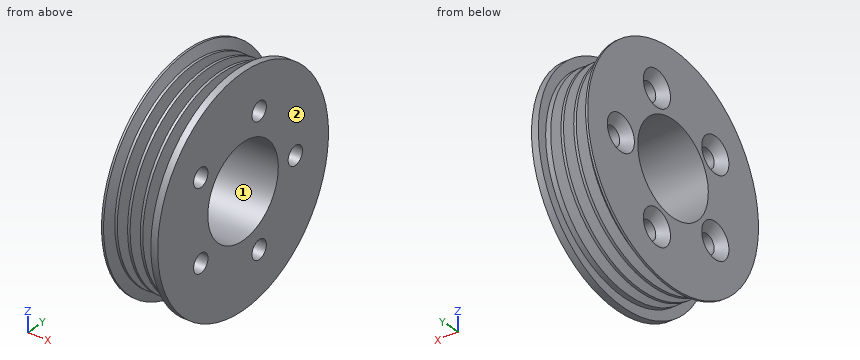
```python
from build123d import *

# Parameters (mm, degrees)
ESCAREADO_PARA_PARAFUSO_COM_CABE_A_ESCAR_D           = 5.5
ESCAREADO_PARA_PARAFUSO_COM_CABE_A_ESCAR_CSINK_D     = 10.4
ESCAREADO_PARA_PARAFUSO_COM_CABE_A_ESCAR_CSINK_ANGLE = 90
PADR_OCIRCULAR1_COUNT                                = 5
ESBO_O5_R                                            = 32.7
ESBO_O5_R_2                                          = 13.5
ESBO_O5_R_3                                          = 2.75
RESSALTO_EXTRUS_O1_DEPTH                             = 2


with BuildPart() as part:
    # Esboço1 → Revolução1 (revolve)
    with BuildSketch(Plane.XY, mode=Mode.PRIVATE) as revolu_o1_sk:
        Polygon((0, 13.5), (16.5, 13.5), (16.5, 29.9), (13, 29.9), (11.9, 24.9), (11.1, 24.9), (10, 29.9), (9.25, 29.9), (8.15, 24.9), (7.35, 24.9), (6.25, 29.9), (5.5, 29.9), (4.4, 24.9), (3.6, 24.9), (2.5, 29.9), (0, 29.9), align=None)
    revolve(revolu_o1_sk.sketch.rotate(Axis((0, 0, 0), (1, 0, 0)), 90), axis=Axis((0, 0, 0), (1, 0, 0)))

    # Escareado para parafuso com cabeça escareada elevada de M51 (through all)
    with Locations(Plane.ZY):
        with Locations((0, 20)):
            escareado_para_parafuso_com_cabe_a_escar = CounterSinkHole(ESCAREADO_PARA_PARAFUSO_COM_CABE_A_ESCAR_D / 2, ESCAREADO_PARA_PARAFUSO_COM_CABE_A_ESCAR_CSINK_D / 2, counter_sink_angle=ESCAREADO_PARA_PARAFUSO_COM_CABE_A_ESCAR_CSINK_ANGLE)

    # PadrãoCircular1: Escareado para parafuso com cabeça escareada elevada de M51 ×5 about axis
    padr_ocircular1_axis = Axis((0, 0, 0), (1, 0, 0))
    for i in range(1, PADR_OCIRCULAR1_COUNT):
        add(escareado_para_parafuso_com_cabe_a_escar.rotate(padr_ocircular1_axis, i * 360 / PADR_OCIRCULAR1_COUNT), mode=Mode.SUBTRACT)

    # Esboço4 → Revolução2 (revolve)
    with BuildSketch(Plane.XY, mode=Mode.PRIVATE) as revolu_o2_sk:
        Polygon((0, 29.9), (0, 32.7), (0.6, 32.7), (1.75, 29.9), align=None)
    revolve(revolu_o2_sk.sketch.rotate(Axis((0, 0, 0), (1, 0, 0)), 90), axis=Axis((0, 0, 0), (1, 0, 0)))

    # Esboço5 → Ressalto-extrusão1 (add)
    with BuildSketch(Plane(origin=(16.5, 0, 0), x_dir=(0, 0, -1), z_dir=(1, 0, 0))):
        with Locations(Location((0, 0, 0), (0, 0, 180))):
            Circle(ESBO_O5_R)
        with Locations(Location((0, 0, 0), (0, 0, 180))):
            Circle(ESBO_O5_R_2, mode=Mode.SUBTRACT)
        with Locations(Location((-11.755705046, -16.180339887, 0), (0, 0, 180))):
            Circle(ESBO_O5_R_3, mode=Mode.SUBTRACT)
        with Locations(Location((11.755705046, -16.180339887, 0), (0, 0, 180))):
            Circle(ESBO_O5_R_3, mode=Mode.SUBTRACT)
        with Locations(Location((19.021130326, 6.180339887, 0), (0, 0, 180))):
            Circle(ESBO_O5_R_3, mode=Mode.SUBTRACT)
        with Locations(Location((0, 20, 0), (0, 0, 180))):
            Circle(ESBO_O5_R_3, mode=Mode.SUBTRACT)
        with Locations(Location((-19.021130326, 6.180339887, 0), (0, 0, 180))):
            Circle(ESBO_O5_R_3, mode=Mode.SUBTRACT)
    extrude(amount=-RESSALTO_EXTRUS_O1_DEPTH)


solid = part.part
```
The model under review builds one solid part; all positions refer to its coordinate system, in mm. Face numbers are marked on the shaded views. Round coordinates to 2 decimals unless told otherwise and drop trailing zeros.
(1) Mouldability with a two-part tool opening along Y and no side actions: class the marked faces 1 and 2 as +Y half, -Y half, draft (parallel to the pull), parting line (faces both ways), or undercut.
(2) We need section A-A on z = 0. Give the number of separate pieces and of enclosed holes in the cut face, and give its area (3 significant figures).
(3) Insertion check: pin 1 (4.5 mm diameter, centred on y = 20, z = 0, fed in from -X); pin 2 (4 mm diameter, centred on x = 8, y = 1.5, fed in from +Z); pin 3 (8 mm diameter, centred on x = 13, y = 21.5, fed in from -Z); pin 4 (5 mm diameter, centred on x = 2.5, y = -21, fed in from +Z). Each pin has a flat end and moves straight along its axis. Give the tip position at first contact, or say it passes through.
(4) Wall thickness on L1, parallel to X at y = -3.5, z = 26; L2, parallel to X at y = -13, z = -21.5; L3, parallel to Z at x = 8, y = 8: over which ranges is each line inside the solid? List them lowest first.
Findings below:
1. face 1: undercut
1. face 2: draft
2. separate pieces: 3
2. enclosed holes: 0
2. area: 405 mm2
3. pin 1: passes through
3. pin 2: stops at z = 29.9
3. pin 3: stops at z = -27.44
3. pin 4: stops at z = 26.34
4. L1: x = 0 to 3.31, 4.69 to 7.06, 8.44 to 10.81, 12.19 to 16.5
4. L2: x = 0 to 3.55, 4.45 to 7.3, 8.2 to 11.05, 11.95 to 16.5
4. L3: z = -23.58 to -21.08, -16.96 to -10.87, 10.87 to 16.96, 21.08 to 23.58
